Verification items for this drawing (mm, ordinates from the low corner). Give positions to 0.01 mm unless a question says otherwise; leave off trailing zeros. Loops run counter-clockwise (first coordinate to the right, second up) from the corner with the lowest first, then second, coordinate; pieces in that order, holes last. Notation, with made-up numbers: M 33,9.5 L 57,9.5 A13 cw 57,16.5 Z; hole C 42.5,54 d1. An arc over 180 degrees is marked long. Use a Markdown table: item, result.
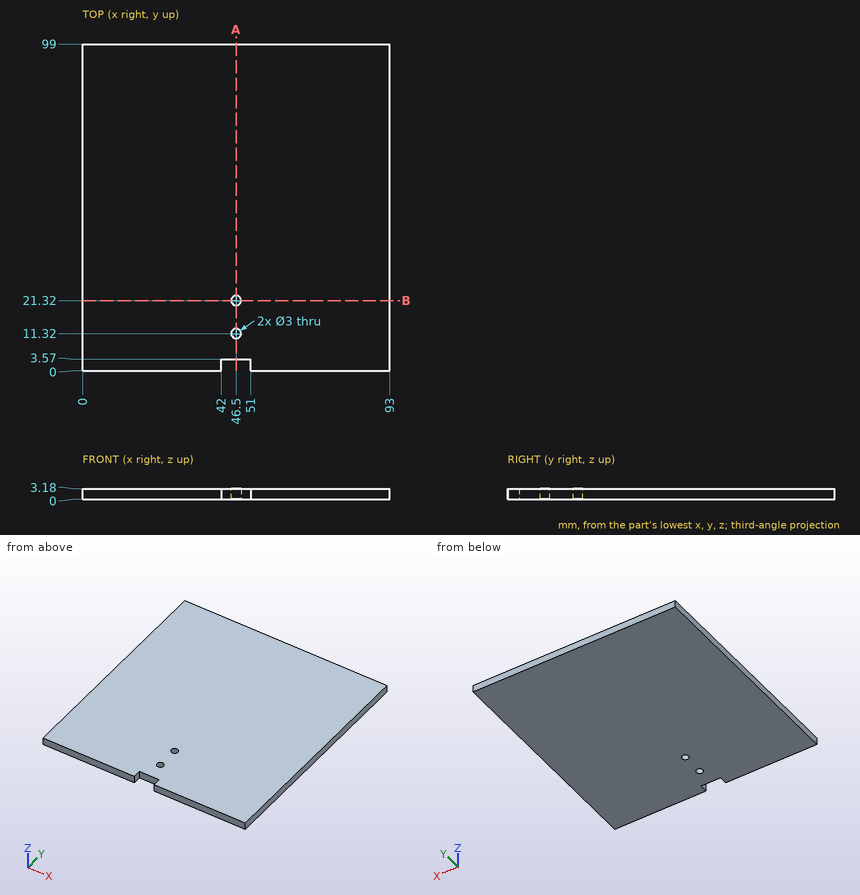
(1) Gauge pin test, flat end, axial feed: P1, Ø1.6, axis at x = 46.5, z = 1, coming from the -Y side. Record the tip position at first contact, or that the pin passes through.
Results below:
| item | result |
|---|---|
| P1 | y = 3.57 |
(2) Material ranges on line 1 (Y direction, x = 46.5, z = 2.1); line 2 (Y direction, x = 49.5, z = 0.4), recorded low to high.
Results below:
| item | result |
|---|---|
| line 1 | 3.57 to 9.82, 12.82 to 19.82, 22.82 to 99 |
| line 2 | 3.57 to 99 |
(3) Cross-section at A-A on x = 46.5. Record the cut outline in (y, z), then the cut area to 3 significant figures.
Results below:
| item | result |
|---|---|
| outline | M 3.57,0 L 9.82,0 L 9.82,3.18 L 3.57,3.18 Z; M 12.82,0 L 19.82,0 L 19.82,3.18 L 12.82,3.18 Z; M 22.82,0 L 99,0 L 99,3.18 L 22.82,3.18 Z |
| area | 284 mm^2 |
(4) Cross-section at B-B on y = 21.32. Record the cut outline in (x, z).
Results below:
| item | result |
|---|---|
| outline | M 0,0 L 45,0 L 45,3.18 L 0,3.18 Z; M 48,0 L 93,0 L 93,3.18 L 48,3.18 Z |
